Autodesk Inventor part; units mm, degrees
ref_plane "YZ Plane" through (0, 0, 0) normal (1, 0, 0) x (0, 1, 0)
ref_plane "XZ Plane" through (0, 0, 0) normal (0, 1, 0) x (-1, 0, 0)
ref_plane "XY Plane" through (0, 0, 0) normal (0, 0, 1) x (1, 0, 0)
sketch "Sketch1" plane through (0, 0, 0) normal (0, 1, 0) x (-1, 0, 0)
  line L0 (0, -19) -> (0, 19) construction
  line L1 (12.9615, 19) -> (-12.9615, 19)
  line L2 (12.9615, -19) -> (-12.9615, -19)
  arc A0 (-12.9615, 19) -> (-12.9615, -19) centre (0, 0) ccw
  arc A1 (12.9615, -19) -> (12.9615, 19) centre (0, 0) ccw
  circle A2 centre (0, 0) radius 6
  dimension "d3" = 12
extrude "Extrusion1" add sketch "Sketch1" along normal blind 6
sketch "Sketch2" plane through (0, 6, 0) normal (0, 1, 0) x (1, 0, 0)
  circle A0 centre (0, 0) radius 14
  dimension "d6" = 28
extrude "Extrusion2" add sketch "Sketch2" along normal blind 4
sketch "Sketch3" plane through (0, 0, 0) normal (0, -1, 0) x (1, 0, 0)
  circle A0 centre (0, 0) radius 11
  dimension "d9" = 22
extrude "Extrusion3" add sketch "Sketch3" along normal blind 6
sketch "Sketch4" plane through (0, -6, 0) normal (0, -1, 0) x (1, 0, 0)
  circle A0 centre (0, 0) radius 6
hole "Hole1" at (0, -6, 0) direction (0, 1, 0) diameter 12 depth 11 tip angle 118
sketch "Sketch5" plane through (0, 10, 0) normal (0, 1, 0) x (1, 0, 0)
  circle A0 centre (0, 0) radius 3.25
  dimension "d19" = 6.5
extrude "Extrusion4" cut sketch "Sketch5" against normal through all
sketch "Sketch6" plane through (0, 6, 0) normal (0, 1, 0) x (1, 0, 0)
  circle A0 centre (0, 0) radius 18 construction
  line L0 (0, 0) -> (12.7279, -12.7279) construction
  line L1 (0, 0) -> (18, 0) construction
  circle A1 centre (12.7279, -12.7279) radius 2.25
  circle A2 centre (12.7279, 12.7279) radius 2.25
  circle A3 centre (-12.7279, 12.7279) radius 2.25
  circle A4 centre (-12.7279, -12.7279) radius 2.25
  dimension "d22" = 36
  dimension "d23" = 45
  dimension "d24" = 4.5
  dimension "d27" = 360
extrude "Extrusion5" cut sketch "Sketch6" against normal through all
properties part number "Testata Superiore"
The listing builds one solid part. Answer for the finished solid, in the listing's coordinates (mm). A direction names the side the tool comes from. Give positions to 0.01 mm unless a question says otherwise; leave off trailing zeros. Order: outer loops, then holes, each group sorted by start corner. A loop starts at its lowest first (then second) coordinate and runs counter-clockwise, first axis right, second up. Notation, with made-up numbers: (5.5, 69) -> (56.5, 69) arc R24 ccw to (56.5, 79) -> close; hole circle Ø4 at (-7.5, 21). An arc over 180 degrees is marked (long way). One line per item, written item: value.
1) Find section B-B, the plane x = 0. Determine the outline of the cut face in (y, z).
Reported:
outline: (-6, -11) -> (0, -11) -> (0, -19) -> (6, -19) -> (6, -14) -> (10, -14) -> (10, -3.25) -> (6.65, -3.25) -> (6, -4.34) -> (6, -6) -> (-6, -6) -> close; (-6, 6) -> (6, 6) -> (6, 4.34) -> (6.65, 3.25) -> (10, 3.25) -> (10, 14) -> (6, 14) -> (6, 19) -> (0, 19) -> (0, 11) -> (-6, 11) -> close
2) Find the intervals of material crossed by line 1 (Z direction, x = 0, y = -0.5); line 2 (X direction, y = 3.5, z = -14); line 3 (X direction, y = 8.65, z = 0), in increasing order.
Reported:
line 1: z = -11 to -6, 6 to 11
line 2: x = -18.25 to -14.58, -10.87 to 10.87, 14.58 to 18.25
line 3: x = -14 to -3.25, 3.25 to 14
3) Find section A-A, the plane z = 0. Determine the outline of the cut face in (x, y), plus the area to 3 significant figures.
Reported:
outline: (-23, 0) -> (-11, 0) -> (-11, -6) -> (-6, -6) -> (-6, 6) -> (-4.34, 6) -> (-3.25, 6.65) -> (-3.25, 10) -> (-14, 10) -> (-14, 6) -> (-23, 6) -> close; (3.25, 6.65) -> (4.34, 6) -> (6, 6) -> (6, -6) -> (11, -6) -> (11, 0) -> (23, 0) -> (23, 6) -> (14, 6) -> (14, 10) -> (3.25, 10) -> close
area: 349 mm^2
4) Determine the mould class of faces 4 (the cylindrical face through (-11.69, 3.042, 14.724)), 5 (the flat face through (3, 10, 3)), 6 (the flat face through (0, 3, 19)) for opening direction Z: pulls with the +Z half, pulls with the -Z half, needs draft (parallel to the pull), parting line crosses it, or undercut.
Reported:
face 4: undercut
face 5: needs draft
face 6: pulls with the +Z half
5) Find section C-C, the plane y = 4.75. Determine the outline of the cut face in (x, z).
Reported:
outline: (-12.96, -19) -> (12.96, -19) arc R23 ccw to (12.96, 19) -> (-12.96, 19) arc R23 ccw to start; hole circle Ø4.5 at (-12.73, -12.73); hole circle Ø4.5 at (-12.73, 12.73); hole circle Ø12 at (0, 0); hole circle Ø4.5 at (12.73, -12.73); hole circle Ø4.5 at (12.73, 12.73)
6) A tool of negligible diameter and unlimited length cuts with its end or side. For faces 1 (the flat face through (11, 0, -4)), 2 (the cylindrical face through (12.932, 7.972, -5.362)), 3 (the cylindrical face through (-11.518, 3.042, -14.625)), from which of +Z, -Z, +X, -X, +Y, -Y can it reach the whole face along a straight path? Write none if from no direction.
Reported:
face 1: -Y
face 2: +Y
face 3: +Y, -Y
7) Flat-ended cylindrical pins translate along their axes: P1, Ø10.5, axis at x = 0, z = 0, coming from the -Y side; P2, Ø7, axis at x = 12.73, z = -12.73, coming from the -Y side; P3, Ø8, axis at y = 5, z = -11, coming from the +X side. Find the tip coordinate at first contact, or state that the pin passes through.
Reported:
P1: stops at y = 6
P2: stops at y = 0
P3: stops at x = 21.91
8) Find section D-D, the plane x = -12. Determine the outline of the cut face in (y, z), plus the area to 3 significant figures.
Reported:
outline: (0, -19) -> (6, -19) -> (6, -14.86) -> (0, -14.86) -> close; (0, -10.6) -> (6, -10.6) -> (6, -7.21) -> (10, -7.21) -> (10, 7.21) -> (6, 7.21) -> (6, 10.6) -> (0, 10.6) -> close; (0, 14.86) -> (6, 14.86) -> (6, 19) -> (0, 19) -> close
area: 235 mm^2
